Input: part model. Units: mm. Frame: model coordinates. A direction names the side the tool comes from. Round coordinates to 2 decimals unless told otherwise and drop trailing zeros. Write each loop counter-clockwise with the first axis right and the second up, starting at its lowest first coordinate (ties: lowest second). Pieces come first, ordered by that corner, then holes. Notation, with made-up numbers: (28, -24) -> (50, -24) arc R15 cw to (50, 2) -> close; hole circle Ø8 at (-5, 48.25). An arc over 180 degrees is marked (long way). Write item = value, one per line. Start each with the question number.
```python
from build123d import *

# Parameters (mm, degrees)
F1_DEPTH = 304.8


with BuildPart() as f1:
    # F0 (on Right) → F1 (new body)
    with BuildSketch(Plane.YZ):
        with BuildLine():
            Line((0, 0), (25.4, 0))
            Line((25.4, 0), (635, 0))
            Line((635, 0), (660.4, 0))
            Line((660.4, 0), (660.4, 69.85))
            Line((660.4, 69.85), (635, 69.85))
            Line((635, 69.85), (508, 69.85))
            ThreePointArc((508, 69.85), (501.120084, 68.473081), (495.3, 64.554436))
            ThreePointArc((495.3, 64.554436), (387.828804, 19.05896), (279.4, 62.222496))
            ThreePointArc((279.4, 62.222496), (273.485985, 66.762175), (266.7, 69.85))
            ThreePointArc((266.7, 69.85), (152.689214, 88.843713), (38.1, 73.726423))
            ThreePointArc((38.1, 73.726423), (28.93043, 67.423949), (25.4, 56.872255))
            Line((25.4, 56.872255), (0, 56.872255))
            Line((0, 56.872255), (0, 0))
        make_face()
    extrude(amount=F1_DEPTH)


solid = f1.part
```
1. Line query: line 1 along Y through (x, z) = (279.5, 50.5); line 2 along Y through (x, z) = (19.5, 31); line 3 along Z through (x, y) = (252, 613). Output: solid intervals per line, ascending.
2. Section C-C (y = 246.5). Output: boundary loops of the cut face in (x, z), then the cut area to 3 significant figures.
3. Section D-D (z = 80). Output: boundary loops of the cut face in (x, y), then the cut area to 3 significant figures.
4. Pin query (flat end, axial travel): P1, Ø12, axis at x = 98, y = 68.5, coming from the +Z side; P2, Ø8, axis at x = 193, z = 64.5, coming from the -Y side; P3, Ø12.5, axis at x = 145, y = 15, coming from the +Z side. Return the tip coordinate at first contact, or that it passes through.
5. Reachability of faces 1 (the cylindrical face through (150.266, 273.576, 66.708)), 2 (the flat face through (150, 585, 69.85)), 3 (the flat face through (150, 13, 56.872)) from +Z, -Z, +X, -X, +Y, -Y: full face, straight path, thin tool, end or side. Return the list, or none.
6. Section A-A (x = 70). Output: boundary loops of the cut face in (y, z), then the cut area to 3 significant figures.
7. Section B-B (z = 46). Output: boundary loops of the cut face in (x, y).
Check sheet entries:
q1.line_1 = 0 to 293.04, 479.3 to 660.4
q1.line_2 = 0 to 326.77, 445.57 to 660.4
q1.line_3 = 0 to 69.85
q2.outline = (0, 0) -> (304.8, 0) -> (304.8, 75.8) -> (0, 75.8) -> close
q2.area = 23,100 mm2
q3.outline = (0, 63.04) -> (304.8, 63.04) -> (304.8, 229.06) -> (0, 229.06) -> close
q3.area = 50,600 mm2
q4.P1 = 82.31
q4.P2 = 25.78
q4.P3 = 56.87
q5.face_1 = +Z, +X, -X
q5.face_2 = +Z, +X, -X, +Y
q5.face_3 = +Z, +X, -X, -Y
q6.outline = (0, 0) -> (660.4, 0) -> (660.4, 69.85) -> (508, 69.85) arc R17.88 ccw to (495.3, 64.55) arc R153.61 cw to (279.4, 62.22) arc R32.82 ccw to (266.7, 69.85) arc R391.58 ccw to (38.1, 73.73) arc R17.53 ccw to (25.4, 56.87) -> (0, 56.87) -> close
q6.area = 40,800 mm2
q7.outline = (0, 0) -> (304.8, 0) -> (304.8, 299.26) -> (0, 299.26) -> close; (0, 473.08) -> (304.8, 473.08) -> (304.8, 660.4) -> (0, 660.4) -> close
